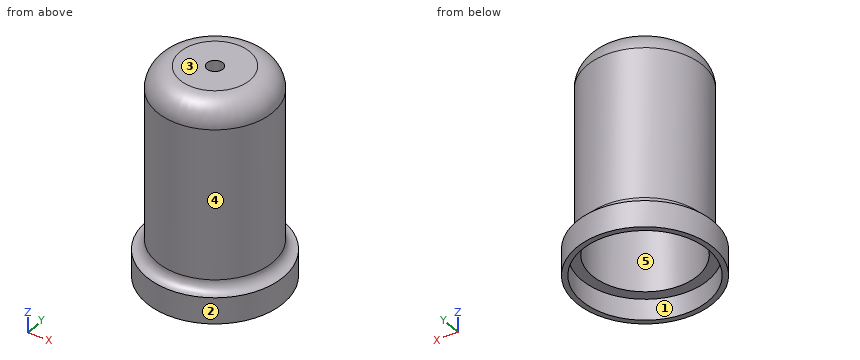
Solid Edge part; units mm, degrees
sketch "Sketch1" plane through (0, 0, 0) normal (0, -1, 0) x (1, 0, 0)
  line L0 (3.25, 0) -> (3.25, 1.25)
  arc A0 (3.25, 1.25) -> (2.75, 1.75) centre (3.25, 1.75) cw
  line L1 (2.75, 1.75) -> (2.75, 8.9106)
  arc A1 (1.6606, 10) -> (2.75, 8.9106) centre (1.6606, 8.9106) cw
  line L2 (1.6606, 10) -> (0, 10)
  line L3 (0, 10) -> (0, 9)
  line L4 (2.5, 9) -> (0, 9)
  line L5 (2.5, 1) -> (2.5, 9)
  line L6 (3, 1) -> (2.5, 1)
  line L7 (3, 0) -> (3, 1)
  line L8 (3, 0) -> (3.25, 0)
revolve "RevolvedProtrusion1" add sketch "Sketch1" angle 360 about axis through (0, 0, 10) along (0, 0, -1)
sketch "Sketch2" plane through (0, 0, 10) normal (0, 0, 1) x (1, 0, 0)
  circle A0 centre (0, 0) radius 0.375
extrude "Cutout1" cut sketch "Sketch2" against normal through all
fillet "Round1" radius 1 1 edges at (-2.5, 0, 9)
CAD build for the part. Positions are in the model's coordinates, mm. Face numbers are marked on the shaded views. A direction names the side the tool comes from. Give positions to 0.01 mm unless a question says otherwise; leave off trailing zeros. Loops run counter-clockwise (first coordinate to the right, second up) from the corner with the lowest first, then second, coordinate; pieces in that order, holes last. Notation, with made-up numbers: (38, 69) -> (66, 69) arc R28 cw to (66, 108) -> close; hole circle Ø11 at (70, 20.25). An arc over 180 degrees is marked (long way). Use a Markdown table: item, result.
1. Wall check: L1, parallel to X at y = 0, z = 4; L2, parallel to Y at x = 0, z = 0.3. Give the ranges that are in metal, low to high. Write a range as [from, to].
Check result:
| item | result |
|---|---|
| L1 | x = [-2.75, -2.5], [2.5, 2.75] |
| L2 | y = [-3.25, -3], [3, 3.25] |
2. Slice it at A-A (y = 0). List the corners of the cut face in (x, z) (3 decimals), plus the area to 3 significant figures.
Check result:
| item | result |
|---|---|
| outline | (-3.25, 0) -> (-3, 0) -> (-3, 1) -> (-2.5, 1) -> (-2.5, 8) arc R1 cw to (-1.5, 9) -> (-0.375, 9) -> (-0.375, 10) -> (-1.661, 10) arc R1.089 ccw to (-2.75, 8.911) -> (-2.75, 1.75) arc R0.5 cw to (-3.25, 1.25) -> close; (0.375, 9) -> (1.5, 9) arc R1 cw to (2.5, 8) -> (2.5, 1) -> (3, 1) -> (3, 0) -> (3.25, 0) -> (3.25, 1.25) arc R0.5 cw to (2.75, 1.75) -> (2.75, 8.911) arc R1.089 ccw to (1.661, 10) -> (0.375, 10) -> close |
| area | 9.53 mm^2 |
3. Slice it at C-C (z = 3). List the corners of the cut face in (x, y), plus the area to 3 significant figures.
Check result:
| item | result |
|---|---|
| outline | circle Ø5.5 at (0, 0); hole circle Ø5 at (0, 0) |
| area | 4.12 mm^2 |
4. Which spindle directions (+Z, -Z, +X, -X, +Y, -Y) get a long thin tool onto all of the face, cutting with end or side? Do the marked faces 1 and 2. Say none if no direction does.
Check result:
| item | result |
|---|---|
| face 1 | -Z |
| face 2 | +Z, -Z |
5. Mould opens along Y. For the marked faces 3, 4 and 5 say: pulls with the +Y half, pulls with the -Y half, needs draft (parallel to the pull), parting line crosses it, or undercut.
Check result:
| item | result |
|---|---|
| face 3 | needs draft |
| face 4 | parting line crosses it |
| face 5 | undercut |
6. Flat gauge pins, fed straight in: pin 1 (2.5 mm diameter, centred on x = 0.5, y = 0, fed in from -Z); pin 2 (1.5 mm diameter, centred on y = -1, z = 7.5, fed in from -X); pin 3 (2 mm diameter, centred on x = 2.5, y = -2, fed in from +Z). Where does each tip first touch, or does it go through?
Check result:
| item | result |
|---|---|
| pin 1 | stops at z = 8.97 |
| pin 2 | stops at x = -2.74 |
| pin 3 | stops at z = 9.86 |
